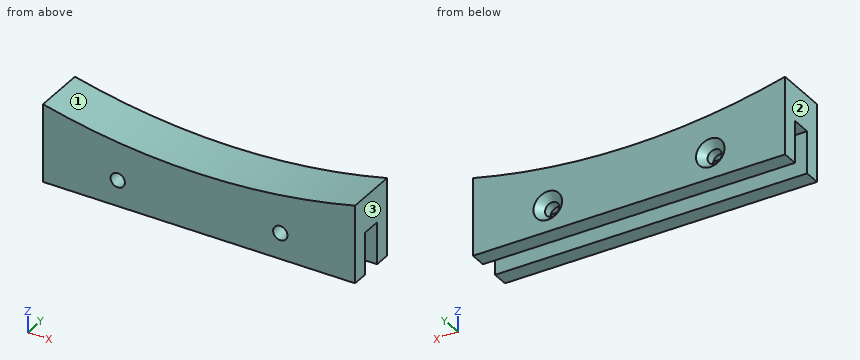
```python
from build123d import *

# Parameters (mm, degrees)
BOSS_EXTRUDE1_DEPTH                             = 4
CSK_FOR_M2_FLAT_HEAD_MACHINE_SCREW1_D           = 2.2
CSK_FOR_M2_FLAT_HEAD_MACHINE_SCREW1_CSINK_D     = 4.4
CSK_FOR_M2_FLAT_HEAD_MACHINE_SCREW1_CSINK_ANGLE = 90
SKETCH9_W                                       = 6.5
SKETCH9_H                                       = 3.05
CUT_EXTRUDE2_DEPTH                              = 50.638694584


with BuildPart() as part:
    # Sketch1 → Boss-Extrude1 (new, symmetric)
    with BuildSketch(Plane(origin=(0, 0, 0), x_dir=(1, 0, 0), z_dir=(0, 1, 0))):
        with BuildLine():
            Line((-24, 0), (24, 0))
            Line((24, 0), (24, -12))
            ThreePointArc((24, -12), (0, -9.077288796), (-24, -12))
            Line((-24, -12), (-24, 0))
        make_face()
    extrude(amount=BOSS_EXTRUDE1_DEPTH, both=True)

    # CSK for M2 Flat Head Machine Screw1 (through all)
    with Locations(Plane(origin=(0, 4, 0), x_dir=(1, 0, 0), z_dir=(0, 1, 0))):
        with Locations((12.5, -4), (-12.5, -4)):
            CounterSinkHole(CSK_FOR_M2_FLAT_HEAD_MACHINE_SCREW1_D / 2, CSK_FOR_M2_FLAT_HEAD_MACHINE_SCREW1_CSINK_D / 2, counter_sink_angle=CSK_FOR_M2_FLAT_HEAD_MACHINE_SCREW1_CSINK_ANGLE)

    # Sketch9 → Cut-Extrude2 (cut, through all)
    with BuildSketch(Plane.ZY.offset(24)):
        with Locations((3.25, 0)):
            Rectangle(SKETCH9_W, SKETCH9_H)
    extrude(amount=-CUT_EXTRUDE2_DEPTH, mode=Mode.SUBTRACT)


solid = part.part
```
The model under review builds one solid part; all positions refer to its coordinate system, in mm. Face numbers are marked on the shaded views. Round coordinates to 2 decimals unless told otherwise and drop trailing zeros. Loops run counter-clockwise (first coordinate to the right, second up) from the corner with the lowest first, then second, coordinate; pieces in that order, holes last.
Item 1: For line 1 (X direction, y = 2.2, z = 4); line 2 (Y direction, x = -16, z = 4.75) (3 decimals); line 3 (X direction, y = -1.75, z = 5), list the stretches that pass through material, from the lowest coordinate up.
Determined:
line 1: x = -24 to -13.6, -11.4 to 11.4, 13.6 to 24
line 2: y = -4 to -1.525, 1.525 to 4
line 3: x = -24 to -12.96, -12.04 to 12.04, 12.96 to 24
Item 2: Take a section at B-B (x = 12.5). Write out the cut boundary in (y, z) (3 decimals), then the cut area to 3 significant figures.
Determined:
outline: (-4, 0) - (-1.525, 0) - (-1.525, 2.9) - (-4, 2.9) - close; (-4, 5.1) - (-1.525, 5.1) - (-1.525, 6.5) - (1.525, 6.5) - (1.525, 5.1) - (2.9, 5.1) - (4, 6.2) - (4, 9.862) - (-4, 9.862) - close; (1.525, 0) - (4, 0) - (4, 1.8) - (2.9, 2.9) - (1.525, 2.9) - close
area: 47.0 mm2
Item 3: Mouldability with a two-part tool opening along X and no side actions: class the marked faces 1, 2 and 3 as released by +X, released by -X, zero draft, split by the parting line, or undercut.
Determined:
face 1: undercut
face 2: released by -X
face 3: released by +X
Item 4: Take a section at A-A (z = 4). Write out the cut boundary in (x, y) (3 decimals).
Determined:
outline: (-24, -4) - (-13.6, -4) - (-13.6, -1.525) - (-24, -1.525) - close; (-24, 1.525) - (-13.6, 1.525) - (-13.6, 2.9) - (-14.7, 4) - (-24, 4) - close; (-11.4, -4) - (11.4, -4) - (11.4, -1.525) - (-11.4, -1.525) - close; (-11.4, 1.525) - (11.4, 1.525) - (11.4, 2.9) - (10.3, 4) - (-10.3, 4) - (-11.4, 2.9) - close; (13.6, -4) - (24, -4) - (24, -1.525) - (13.6, -1.525) - close; (13.6, 1.525) - (24, 1.525) - (24, 4) - (14.7, 4) - (13.6, 2.9) - close
Item 5: Take a section at C-C (y = 2). Write out the cut boundary in (x, z), then the cut area to 3 significant figures.
Determined:
outline: (-24, 0) - (24, 0) - (24, 12) arc R100 cw to (-24, 12) - close; hole circle Ø2.2 at (-12.5, 4); hole circle Ø2.2 at (12.5, 4)
area: 475 mm2
Item 6: Clearance check with flat-ended pins moving along their axes: pin 1 Ø1.8 at (x, z) = (-12.5, 4) entering from +Y; pin 2 Ø3.5 at (x, z) = (12.5, 4) entering from +Y; pin 3 Ø3 at (y, z) = (-1.5, 6) entering from -X. State where each tip first meets the part, or that it passes through.
Determined:
pin 1: passes through
pin 2: stops at y = 3.55
pin 3: stops at x = -24
Item 7: Take a section at D-D (z = 10). Write out the cut boundary in (x, y).
Determined:
outline: (-24, -4) - (-13.55, -4) - (-13.55, 4) - (-24, 4) - close; (13.55, -4) - (24, -4) - (24, 4) - (13.55, 4) - close
